Autodesk Inventor part; units mm, degrees
ref_plane "YZ Plane" through (0, 0, 0) normal (1, 0, 0) x (0, 1, 0)
ref_plane "XZ Plane" through (0, 0, 0) normal (0, 1, 0) x (-1, 0, 0)
ref_plane "XY Plane" through (0, 0, 0) normal (0, 0, 1) x (1, 0, 0)
sketch "Skizze1" plane through (0, 0, 0) normal (0, 1, 0) x (-1, 0, 0)
  line L0 (0, 0) -> (0, 6.5)
  line L1 (0, 6.5) -> (-20, 6.5)
  line L2 (-20, 6.5) -> (-20, 5)
  line L3 (-20, 5) -> (-22, 5)
  line L4 (-22, 5) -> (-22, 6.5)
  line L5 (-22, 6.5) -> (-50.5, 6.5)
  line L6 (-50.5, 6.5) -> (-50.5, 0)
  line L7 (-50.5, 0) -> (0, 0)
  dimension "d0" = 13
  dimension "d1" = 20
  dimension "d2" = 2
  dimension "d3" = 28.5
  dimension "d4" = 10
revolve "Umdrehung1" add sketch "Skizze1" angle 360 about axis through (50.5, 0, 0) along (-1, 0, 0)
sketch "Skizze2" plane through (0, 0, 0) normal (-1, 0, 0) x (0, 0, 1)
  circle A0 centre (0, 0) radius 6.5
  point P0 (0, 0)
hole "Bohrung1" at (0, 0, 0) direction (1, 0, 0) diameter 6 end through all
fillet "Rundung1" radius 0.6 2 edges at (0, 0, -6.5) (50.5, 0, -6.5)
properties part number "204 Welle" material "Aluminum 6061-AHC"
Read the model definition and answer for the solid it produces. Units are mm, in the model's axes. A direction names the side the tool comes from. Coordinates: 2 decimals unless noted, no trailing zeros. Write each loop counter-clockwise with the first axis right and the second up, starting at its lowest first coordinate (ties: lowest second). Pieces come first, ordered by that corner, then holes. Notation, with made-up numbers: M 62.25,1.25 L 91.25,1.25 A22 ccw 91.25,30.25 Z; hole C 35.5,-8.75 d1. An arc over 180 degrees is marked long. Use a Markdown table: item, result.
Q1. Determine the mould class of faces 3 (the face through (50.5, 1, -3)), 4 (the face through (26, 0, -3)), 5 (the face through (21.01, 4.88, -1.08)) for opening direction Y: released by +Y, released by -Y, zero draft, split by the parting line, or undercut.
Answer block:
| item | result |
|---|---|
| face 3 | zero draft |
| face 4 | undercut |
| face 5 | split by the parting line |
Q2. The part is cut by section C-C, the plane x = 30. Write down the section's boundary in (y, z), then the cut area to 3 significant figures.
Answer block:
| item | result |
|---|---|
| outline | C 0,0 d13; hole C 0,0 d6 |
| area | 104 mm2 |
Q3. Each of these flat-tipped pins is pushed along its axis until it touches: pin 1 Ø1.5 at (x, z) = (22, -1) entering from -Y; pin 2 Ø3.5 at (y, z) = (0, 0) entering from +X; pin 3 Ø6 at (x, z) = (13.5, 5) entering from -Y. Where does it stop, or does it pass through?
Answer block:
| item | result |
|---|---|
| pin 1 | stops at y = -6.5 |
| pin 2 | passes through |
| pin 3 | stops at y = -6.18 |
Q4. Straight lines are drawn through the part: L1, parallel to Y at x = 28.5, z = 0; L2, parallel to X at y = 2.75, z = -5; L3, parallel to Z at x = 9, y = 2. For each, find the intervals that lie inside material, in ascending order. Write a range as [from, to].
Answer block:
| item | result |
|---|---|
| L1 | y = [-6.5, -3], [3, 6.5] |
| L2 | x = [0, 20], [22, 50.5] |
| L3 | z = [-6.18, -2.24], [2.24, 6.18] |
Q5. Which of the six approach directions +Z, -Z, +X, -X, +Y, -Y give full straight-line access (tool end or side, diameter ignored) to faces 1 (the face through (22, -5, 2)), 2 (the face through (36.145, 3.955, -5.158))?
Answer block:
| item | result |
|---|---|
| face 1 | none |
| face 2 | +X, -X |
Q6. The part is cut by section A-A, the plane z = 0. Write down the section's boundary in (x, y), then the cut area to 3 significant figures.
Answer block:
| item | result |
|---|---|
| outline | M 0,-5.9 A0.6 ccw 0.6,-6.5 L 20,-6.5 L 20,-5 L 22,-5 L 22,-6.5 L 49.9,-6.5 A0.6 ccw 50.5,-5.9 L 50.5,-3 L 0,-3 Z; M 0,3 L 50.5,3 L 50.5,5.9 A0.6 ccw 49.9,6.5 L 22,6.5 L 22,5 L 20,5 L 20,6.5 L 0.6,6.5 A0.6 ccw 0,5.9 Z |
| area | 347 mm2 |
